```python
from build123d import *

# Parameters (mm, degrees)
PAD_DEPTH       = 20
POCKET_DEPTH    = 5
POCKET001_DEPTH = 5


with BuildPart() as part:
    # Sketch → Pad (new body)
    with BuildSketch(Plane.XY):
        Polygon((-30.124981, 30.287271), (23.4375, 30.287271), (52.34375, 3.437501), (32.656242, -29.0625), (32.656242, -49.867283), (-20.964462, -49.867283), (-20.964462, -28.68358), (-50.354469, -10.171695), align=None)
    extrude(amount=PAD_DEPTH)

    # Sketch001 (on Face10 of Pad) → Pocket (cut)
    with BuildSketch(Plane.XY.offset(20)):
        Polygon((-25.927446, 17.441479), (-7.606405, 17.441479), (-7.606405, -6.032361), (-27.454205, -6.032361), align=None)
        Polygon((13.768158, 16.868948), (27.127254, 16.868948), (28.081469, -5.841516), (12.050557, -6.414047), align=None)
    extrude(amount=-POCKET_DEPTH, mode=Mode.SUBTRACT)

    # Sketch002 (on Face5 of Pocket) → Pocket001 (cut)
    with BuildSketch(Plane.XY.offset(20)):
        Polygon((0, -10.881702), (-10.45758, -25.686424), (12.034194, -24.5476), align=None)
    extrude(amount=-POCKET001_DEPTH, mode=Mode.SUBTRACT)


solid = part.part
```
CAD build for the part. Positions are in the model's coordinates, mm. A direction names the side the tool comes from. Round coordinates to 2 decimals unless told otherwise and drop trailing zeros. Order: outer loops, then holes, each group sorted by start corner. A loop starts at its lowest first (then second) coordinate and runs counter-clockwise, first axis right, second up. Notation, with made-up numbers: (-25.5, 20) - (1.5, 20) arc R30 ccw to (1.5, 46) - close; hole circle Ø11 at (19, 5.25). An arc over 180 degrees is marked (long way). Answer in a Markdown table with one row per item. Add a question column.
(1) Probe L1, parallel to Z at x = -25, y = -5.5; L2, parallel to X at y = 0.5, z = 16; L3, parallel to X at y = 5.5, z = 19. List the from-to ranges inside material, lowest first. Write a range as [from, to].
(2) 3-axis set-ups, long thin cutter, end or side, ignore diameter. For faces 5 (the face through (27.598, 5.673, 17.535)), 6 (the face through (-20.964, -39, 10)), 7 (the face through (6, -49.867, 10)): which of +Z, -Z, +X, -X, +Y, -Y reach the whole face in a straight line?
(3) Mould opens along X. For faces 1 (the face through (42.64, -12.58, 9.86)), 2 (the face through (2, -9, 0)), 3 (the face through (-40.381, 9.775, 9.86)), 4 (the face through (6.1, -17.81, 17.54)) say: +X half, -X half, draft (parallel to the pull), parting line (faces both ways), or undercut.
(4) Band-saw the part on C-C on y = -39. List the corners of the cut face in (x, z), and give its area (3 significant figures).
(5) Band-saw the part on A-A on z = 13.75. List the corners of the cut face in (x, y).
(6) Band-saw the part on B-B on x = 1.5. List the corners of the cut face in (y, z), and give its area (3 significant figures).
(7) Band-saw the part on D-D on y = 9.5. List the corners of the cut face in (x, z).
(8) Drop flat-ended pins along their axis: pin 1 Ø2 at (x, y) = (-38, -19.5) entering from -Z; pin 2 Ø4 at (y, z) = (9.5, 18) entering from -X; pin 3 Ø8 at (y, z) = (21, 3.5) entering from -X; pin 4 Ø3 at (y, z) = (-18.5, 11) entering from -X. Give the stop position or say it passes through.
Data:
| question | item | result |
|---|---|---|
| 1 | L1 | z = [0, 15] |
| 1 | L2 | x = [-45.02, -27.03], [-7.61, 12.56], [27.82, 50.56] |
| 1 | L3 | x = [-42.52, -26.7], [-7.61, 12.93], [27.6, 50.12] |
| 2 | face 5 | +Z |
| 2 | face 6 | +Z, -Z, -X, -Y |
| 2 | face 7 | +Z, -Z, +X, -X, -Y |
| 3 | face 1 | +X half |
| 3 | face 2 | draft |
| 3 | face 3 | -X half |
| 3 | face 4 | undercut |
| 4 | outline | (-20.96, 0) - (32.66, 0) - (32.66, 20) - (-20.96, 20) - close |
| 4 | area | 1,070 mm^2 |
| 5 | outline | (-50.35, -10.17) - (-20.96, -28.68) - (-20.96, -49.87) - (32.66, -49.87) - (32.66, -29.06) - (52.34, 3.44) - (23.44, 30.29) - (-30.12, 30.29) - close |
| 6 | outline | (-49.87, 0) - (30.29, 0) - (30.29, 20) - (-12.59, 20) - (-12.59, 15) - (-25.08, 15) - (-25.08, 20) - (-49.87, 20) - close |
| 6 | area | 1,540 mm^2 |
| 7 | outline | (-40.52, 0) - (45.82, 0) - (45.82, 20) - (27.44, 20) - (27.44, 15) - (13.22, 15) - (13.22, 20) - (-7.61, 20) - (-7.61, 15) - (-26.44, 15) - (-26.44, 20) - (-40.52, 20) - close |
| 8 | pin 1 | passes through |
| 8 | pin 2 | stops at x = -41.52 |
| 8 | pin 3 | stops at x = -36.77 |
| 8 | pin 4 | stops at x = -39.51 |
